```python
from build123d import *

# Parameters (mm, degrees)
BOSS_EXTRUDE1_DEPTH = 1.6
SKETCH2_R           = 1.4
CUT_EXTRUDE1_DEPTH  = 1.6
SKETCH3_R           = 5
CUT_EXTRUDE2_DEPTH  = 1.6
SKETCH4_R           = 1.6
CUT_EXTRUDE3_DEPTH  = 10


with BuildPart() as part:
    # Sketch1 → Boss-Extrude1 (new body)
    with BuildSketch(Plane.XY):
        Polygon((32, 28), (36, 24), (36, -24), (32, -28), (-32, -28), (-36, -24), (-36, 24), (-32, 28), align=None)
    extrude(amount=BOSS_EXTRUDE1_DEPTH)

    # Sketch2 → Cut-Extrude1 (cut)
    with BuildSketch(Plane.XY.offset(1.6)):
        with Locations((-31, 23)):
            Circle(SKETCH2_R)
        with Locations((31, 23)):
            Circle(SKETCH2_R)
        with Locations((-31, -23)):
            Circle(SKETCH2_R)
        with Locations((31, -23)):
            Circle(SKETCH2_R)
    extrude(amount=-CUT_EXTRUDE1_DEPTH, mode=Mode.SUBTRACT)

    # Sketch3 → Cut-Extrude2 (cut)
    with BuildSketch(Plane.XY.offset(1.6)):
        with Locations((25.4, -13.5)):
            Circle(SKETCH3_R)
    extrude(amount=-CUT_EXTRUDE2_DEPTH, mode=Mode.SUBTRACT)

    # Sketch4 → Cut-Extrude3 (cut)
    with BuildSketch(Plane.XY.offset(1.6)):
        with Locations((-19.9, -24.4)):
            Circle(SKETCH4_R)
        with Locations((-9.75, -24.698906537)):
            Circle(SKETCH4_R)
        with Locations((-2.55, -24.4)):
            Circle(SKETCH4_R)
        with Locations((7.6, -24.4)):
            Circle(SKETCH4_R)
        with Locations((-32.4, -17.075)):
            Circle(SKETCH4_R)
        with Locations((-32.4, -6.925)):
            Circle(SKETCH4_R)
    extrude(amount=-CUT_EXTRUDE3_DEPTH, mode=Mode.SUBTRACT)


solid = part.part
```
For this review, take the finished solid that the model builds, in its own axes (mm). Round coordinates to 2 decimals unless told otherwise and drop trailing zeros. Write each loop counter-clockwise with the first axis right and the second up, starting at its lowest first coordinate (ties: lowest second). Pieces come first, ordered by that corner, then holes. Notation, with made-up numbers: (-2.5, 16) -> (10.5, 16) arc R25 cw to (10.5, 52) -> close; hole circle Ø6 at (-23.5, -16.5). An arc over 180 degrees is marked (long way). One line per question, with ' | ' between items. Start each with the question number.
(1) Add section D-D, the plane z = 1.1. Give the number of separate pieces and of enclosed holes in the cut face, plus the area to 3 significant figures.
(2) Add section B-B, the plane x = 25.4. Write out the cut boundary in (y, z), plus the area to 3 significant figures.
(3) Mouldability with a two-part tool opening along Y and no side actions: class faces 1 (the face through (0, -28, 1)), 2 (the face through (1, 0, 0)), 3 (the face through (30.019, -15.415, 0.811)) as released by +Y, released by -Y, zero draft, split by the parting line, or undercut.
(4) For line 1 along Y through (x, z) = (-31, 1.15); line 2 along X through (y, z) = (-25, 0.1); line 3 along Y through (x, z) = (-19.5, 0.45), list the stretches that pass through material, from the lowest coordinate up. Write a range as from..to.
(5) Add section C-C, the plane y = -13.5. Write out the cut boundary in (x, z).
(6) Add section A-A, the plane y = 23. Write out the cut boundary in (x, z), plus the area to 3 significant figures.
Answer list:
1) separate pieces: 1 | enclosed holes: 11 | area: 3,850 mm²
2) outline: (-28, 0) -> (-18.5, 0) -> (-18.5, 1.6) -> (-28, 1.6) -> close; (-8.5, 0) -> (28, 0) -> (28, 1.6) -> (-8.5, 1.6) -> close | area: 73.6 mm²
3) face 1: released by -Y | face 2: zero draft | face 3: undercut
4) line 1: -28..-24.4, -21.6..-17.85, -16.3..-7.7, -6.15..21.6, 24.4..28 | line 2: -35..-21.38, -18.42..-11.32, -8.18..-4.03, -1.07..6.12, 9.08..35 | line 3: -28..-25.95, -22.85..28
5) outline: (-36, 0) -> (20.4, 0) -> (20.4, 1.6) -> (-36, 1.6) -> close; (30.4, 0) -> (36, 0) -> (36, 1.6) -> (30.4, 1.6) -> close
6) outline: (-36, 0) -> (-32.4, 0) -> (-32.4, 1.6) -> (-36, 1.6) -> close; (-29.6, 0) -> (29.6, 0) -> (29.6, 1.6) -> (-29.6, 1.6) -> close; (32.4, 0) -> (36, 0) -> (36, 1.6) -> (32.4, 1.6) -> close | area: 106 mm²
